Part print with two shaded views. Sizes in mm from the minimum x, y, z corner. A direction names the side the tool comes from. Round coordinates to 2 decimals unless told otherwise and drop trailing zeros. Loops run counter-clockwise (first coordinate to the right, second up) from the corner with the lowest first, then second, coordinate; pieces in that order, holes last. Notation, with made-up numbers: (-27, 56.25) -> (-18, 56.25) arc R25 cw to (-18, 70.25) -> close; hole circle Ø2 at (69.5, -18). An arc over 180 degrees is marked (long way). Use a Markdown table: item, result. Add a question column.
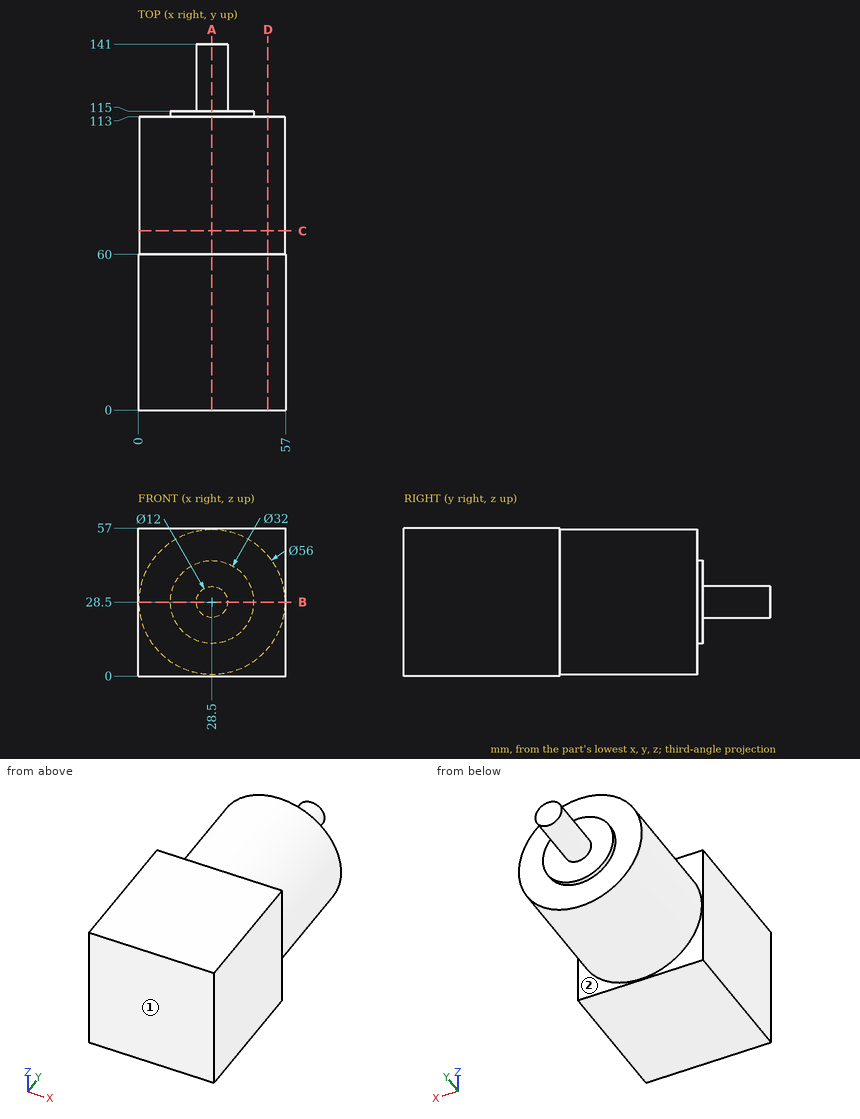
1) Cut at C-C on y = 69. Write the cut outline in (x, z), and give its area (3 significant figures).
2) Pin check, flat tips, straight feed: pin 1 Ø2 at (x, y) = (34.5, 35.5) entering from -Z; pin 2 Ø2 at (x, y) = (35, 119) entering from +Z; pin 3 Ø12 at (y, z) = (85, 18) entering from -X; pin 4 Ø6 at (x, y) = (28.5, 76.5) entering from -Z. Stop position of each tip, or through.
3) Cut at B-B on z = 28.5. Write the cut outline in (x, y).
4) Cut at D-D on x = 50. Write the cut outline in (y, z), and give its area (3 significant figures).
5) Wall check: probe 1 along Y at (x, z) = (15, 46.5); probe 2 along Y at (x, z) = (3, 8.5); probe 3 along Z at (x, y) = (46, 97.5). Give the ranges that are in metal, low to high. Write a range as from..to.
6) Tool access for the marked faces 1 and 2: list every direction of +Z, -Z, +X, -X, +Y, -Y with a clear straight run to the whole face (end or side of a thin tool).
7) Cut at A-A on x = 28.5. Write the cut outline in (y, z).
Established:
| question | item | result |
|---|---|---|
| 1 | outline | circle Ø56 at (28.5, 28.5) |
| 1 | area | 2,460 mm^2 |
| 2 | pin 1 | stops at z = 0 |
| 2 | pin 2 | stops at z = 30.9 |
| 2 | pin 3 | stops at x = 0.86 |
| 2 | pin 4 | stops at z = 0.5 |
| 3 | outline | (0, 0) -> (57, 0) -> (57, 60) -> (56.5, 60) -> (56.5, 113) -> (44.5, 113) -> (44.5, 115) -> (34.5, 115) -> (34.5, 141) -> (22.5, 141) -> (22.5, 115) -> (12.5, 115) -> (12.5, 113) -> (0.5, 113) -> (0.5, 60) -> (0, 60) -> close |
| 4 | outline | (0, 0) -> (60, 0) -> (60, 10.56) -> (113, 10.56) -> (113, 46.44) -> (60, 46.44) -> (60, 57) -> (0, 57) -> close |
| 4 | area | 5,320 mm^2 |
| 5 | probe 1 | y = 0..113 |
| 5 | probe 2 | y = 0..60 |
| 5 | probe 3 | z = 6.64..50.36 |
| 6 | face 1 | +Z, -Z, +X, -X, -Y |
| 6 | face 2 | +Y |
| 7 | outline | (0, 0) -> (60, 0) -> (60, 0.5) -> (113, 0.5) -> (113, 12.5) -> (115, 12.5) -> (115, 22.5) -> (141, 22.5) -> (141, 34.5) -> (115, 34.5) -> (115, 44.5) -> (113, 44.5) -> (113, 56.5) -> (60, 56.5) -> (60, 57) -> (0, 57) -> close |
